Geometry check sheet. Reference: the model listing, model coordinates, mm. Face numbers are marked on the shaded views. A direction names the side the tool comes from. Coordinates: 2 decimals unless noted, no trailing zeros. Order: outer loops, then holes, each group sorted by start corner. A loop starts at its lowest first (then second) coordinate and runs counter-clockwise, first axis right, second up. Notation, with made-up numbers: (63.25, -36.5) -> (122.25, -36.5) arc R16 cw to (122.25, -19.5) -> close; hole circle Ø9 at (27.5, 48). An arc over 180 degrees is marked (long way). Answer in a Markdown table with one row per item. Add a question column.
```python
from build123d import *

# Parameters (mm, degrees)
F0_W     = 9.8
F0_H     = 9.8
F0_R     = 2.5
F1_DEPTH = 1.5
F2_DEPTH = 12
F3_R     = 2.5


with BuildPart() as f1:
    # F0 (on Front) → F1 (new body, symmetric)
    with BuildSketch(Plane.XZ):
        Rectangle(F0_W, F0_H)
        Circle(F0_R, mode=Mode.SUBTRACT)
        Circle(F0_R)
    extrude(amount=F1_DEPTH, both=True)

    # F0 (on Front) → F2 (join)
    with BuildSketch(Plane.XZ):
        Circle(F0_R)
    extrude(amount=F2_DEPTH)

    # F3
    f3_edges = [f1.edges().sort_by_distance(p)[0] for p in [
        (-2.5, -12, 0),
    ]]
    fillet(f3_edges, radius=F3_R)


solid = f1.part
```
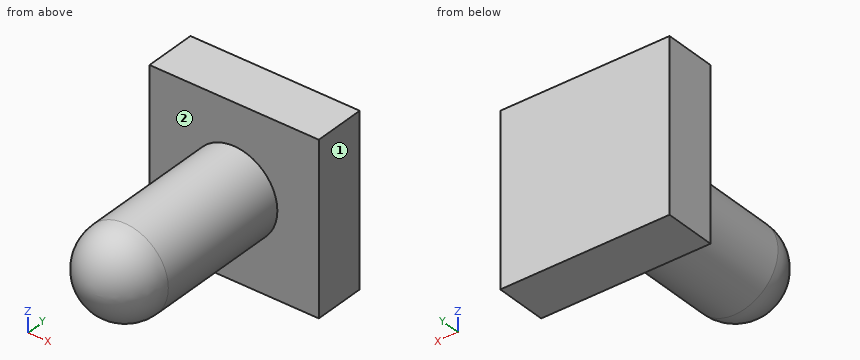
(1) Scan lines: line 1 along Y through (x, z) = (-2, 1.75); line 2 along Z through (x, y) = (0, -3). Record each from-to range of solid material in increasing order.
(2) Cross-section at B-B (z = -2). Enter the section's corners in (x, y).
(3) Go/stop test with flat-tipped pins: P1, Ø5, axis at x = -1, y = -2.5, coming from the +Z side; P2, Ø3, axis at x = 1.5, z = 1.5, coming from the -Y side; P3, Ø3, axis at x = -0.5, y = -10, coming from the +Z side; P4, Ø1.5, axis at y = -6, z = -4, coming from the +X side. Record where each tip stops, or that it passes through.
(4) Access from +Z, -Z, +X, -X, +Y, -Y to the whole of each face (thin tool, end or side, straight path). Record for the marked faces 1 and 2.
(5) Cross-section at A-A (x = 0). Enter the section's corners in (y, z).
(6) Cross-section at C-C (y = -9). Enter the section's corners in (x, z), plus the area to 3 significant figures.
(7) Cross-section at D-D (z = -3). Enter the section's corners in (x, y), plus the area to 3 significant figures.
Checks:
| question | item | result |
|---|---|---|
| 1 | line 1 | -1.5 to 1.5 |
| 1 | line 2 | -2.5 to 2.5 |
| 2 | outline | (-4.9, -1.5) -> (-1.5, -1.5) -> (-1.5, -9.5) arc R1.5 ccw to (1.5, -9.5) -> (1.5, -1.5) -> (4.9, -1.5) -> (4.9, 1.5) -> (-4.9, 1.5) -> close |
| 3 | P1 | z = 4.9 |
| 3 | P2 | y = -11.92 |
| 3 | P3 | z = 2.5 |
| 3 | P4 | through |
| 4 | face 1 | +Z, -Z, +X, +Y, -Y |
| 4 | face 2 | -Y |
| 5 | outline | (-9.5, -2.5) -> (-1.5, -2.5) -> (-1.5, -4.9) -> (1.5, -4.9) -> (1.5, 4.9) -> (-1.5, 4.9) -> (-1.5, 2.5) -> (-9.5, 2.5) arc R2.5 ccw to start |
| 6 | outline | circle Ø5 at (0, 0) |
| 6 | area | 19.6 mm² |
| 7 | outline | (-4.9, -1.5) -> (4.9, -1.5) -> (4.9, 1.5) -> (-4.9, 1.5) -> close |
| 7 | area | 29.4 mm² |
